Print and shaded views of the part. All mm, measured from the part's lowest x, y and z. A direction names the side the tool comes from. Give positions to 0.01 mm unless a question says otherwise; leave off trailing zeros. Loops run counter-clockwise (first coordinate to the right, second up) from the corner with the lowest first, then second, coordinate; pieces in that order, holes last.
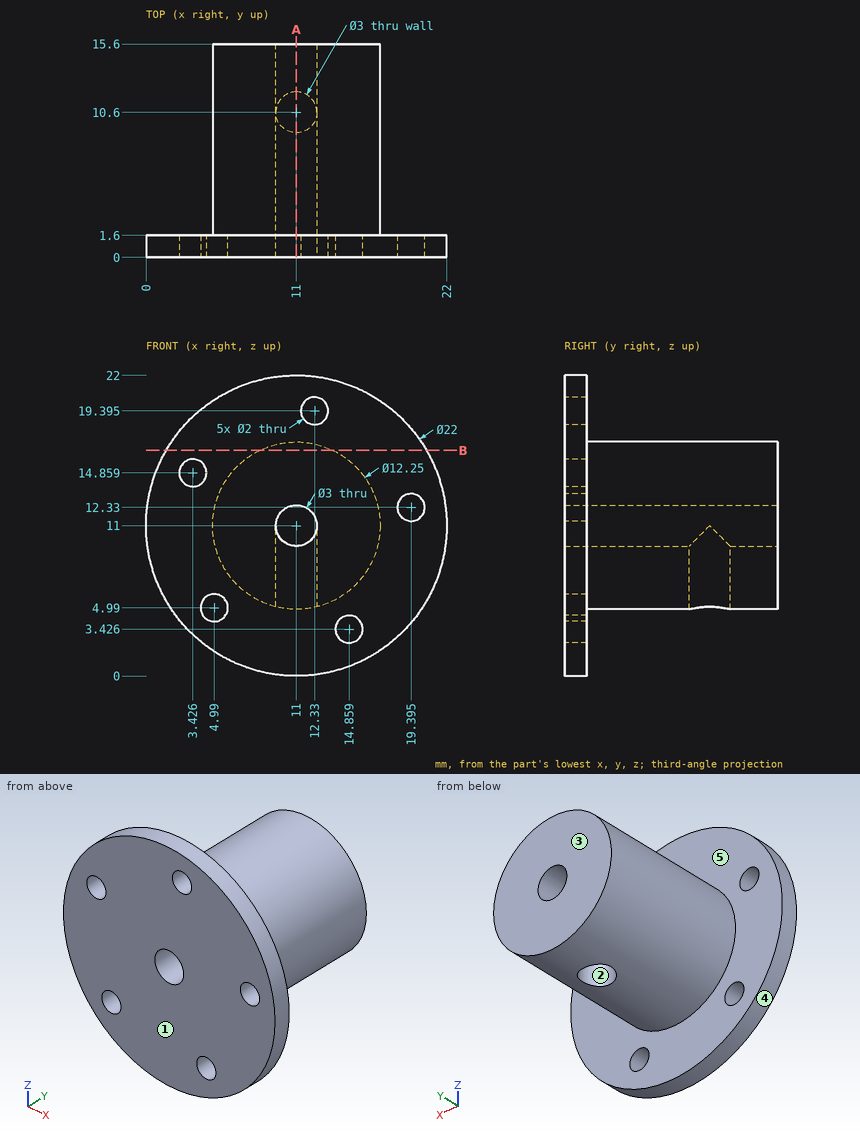
1. Tool access for the marked faces 4 and 5: list every direction of +Z, -Z, +X, -X, +Y, -Y with a clear straight run to the whole face (end or side of a thin tool).
Responses:
face 4: +Y, -Y
face 5: +Y
2. Saw through at B-B, the plane z = 16.5. List the corners of the cut face in (x, y) (1 decimal), and give its area (3 significant figures).
Responses:
outline: (1.5, 0) - (20.5, 0) - (20.5, 1.6) - (13.7, 1.6) - (13.7, 15.6) - (8.3, 15.6) - (8.3, 1.6) - (1.5, 1.6) - close
area: 106 mm2
3. Drop flat-ended pins along their axis: pin 1 (3 mm diameter, centred on x = 14.86, z = 3.43, fed in from -Y); pin 2 (1.6 mm diameter, centred on x = 19.4, z = 12.33, fed in from +Y); pin 3 (4 mm diameter, centred on x = 2.5, y = 2.5, fed in from -Z) (1 decimal); pin 4 (1 mm diameter, centred on x = 14, y = 10, fed in from +Z). Give the stop position or say it passes through.
Responses:
pin 1: stops at y = 0
pin 2: passes through
pin 3: stops at z = 2.3
pin 4: stops at z = 16.59
4. Pull direction Y, two halves, no side cores. Call the marked faces 1, 2 and 3: released by +Y, released by -Y, zero draft, split by the parting line, or undercut.
Responses:
face 1: released by -Y
face 2: undercut
face 3: released by +Y
5. Probe line 1 along X through (y, z) = (12, 11) (1 decimal); line 2 along Y through (x, z) = (2.75, 6.75); line 3 along Y through (x, z) = (11, 8). List the from-to ranges inside material, lowest first.
Responses:
line 1: x = 4.9 to 9.5, 12.5 to 17.1
line 2: y = 0 to 1.6
line 3: y = 0 to 9.1, 12.1 to 15.6
6. Saw through at A-A, the plane x = 11. List the corners of the cut face in (y, z) (1 decimal).
Responses:
outline: (0, 0) - (1.6, 0) - (1.6, 4.9) - (9.1, 4.9) - (9.1, 9.5) - (0, 9.5) - close; (0, 12.5) - (15.6, 12.5) - (15.6, 17.1) - (1.6, 17.1) - (1.6, 22) - (0, 22) - close; (12.1, 4.9) - (15.6, 4.9) - (15.6, 9.5) - (12.1, 9.5) - close
